Part model, mm, in its own coordinate system. A direction names the side the tool comes from. Round coordinates to 2 decimals unless told otherwise and drop trailing zeros. Write each loop counter-clockwise with the first axis right and the second up, starting at its lowest first coordinate (ties: lowest second). Pieces come first, ordered by that corner, then holes. Notation, with made-up numbers: M -11,-10 L 46,-10 A18 ccw 46,5 Z; hole C -28,89.25 d4. An arc over 180 degrees is marked long. Use a Markdown table: item, result. Add a question column.
1) Which spindle directions (+Z, -Z, +X, -X, +Y, -Y) get a long thin tool onto all of the face, cutting with end or side? Do faces 1 (the face through (16, 4.826, 20)), 2 (the face through (33.018, -22.918, 7.776)). Say none if no direction does.
2) Two-plate mould, pull along X, no slides. Class faces 3 (the face through (33.7, 22.8, 7.8)), 4 (the face through (-14.277, 0.559, 20.398)), 5 (the face through (16, -4.826, 20)), 6 (the face through (11, -11, 40.234)): released by +X, released by -X, zero draft, split by the parting line, or undercut.
3) Slice it at B-B on x = 52. Write the cut outline in (y, z).
4) Slice it at A-A on z = 6.5. Give the number of separate pieces and of enclosed holes in the cut face, plus the area to 3 significant figures.
5) Wall check: probe 1 along Y at (x, z) = (0, 12.5) (1 decimal); probe 2 along X at (y, z) = (1, 8.5); probe 3 along X at (y, z) = (-5, 25). Give the ranges that are in metal, low to high.
6) Drop flat-ended pins along their axis: P1, Ø12, axis at y = -11.5, z = 10, coming from the -X side; P2, Ø6, axis at x = 57.5, y = 12.5, coming from the +Z side; P3, Ø12, axis at x = 60.5, z = 6, coming from the +Y side; P4, Ø16.5, axis at x = 53.975, y = 0, coming from the -Z side. Give the stop position or say it passes through.
```python
from build123d import *

# Parameters (mm, degrees)
F1_DEPTH = 40.2336
F2_R     = 10.16
F3_DEPTH = 15.7734
F5_DEPTH = 40.2346
F6_R     = 3.302


with BuildPart() as f1:
    # F0 (on Top) → F1 (new body)
    with BuildSketch(Plane.XY):
        with BuildLine():
            ThreePointArc((9.512184, -26.945296), (23.327466, -16.503332), (28.575, 0))
            ThreePointArc((28.575, 0), (23.327466, 16.503332), (9.512184, 26.945296))
            ThreePointArc((9.512184, 26.945296), (-28.575, 0), (9.512184, -26.945296))
        make_face()
    extrude(amount=F1_DEPTH)

    # F2 (on Top) + F0 (on Top) → F3 (join)
    with BuildSketch(Plane.XY):
        with BuildLine():
            ThreePointArc((57.191927, -18.776418), (68.538395, -12.280473), (73.025, 0))
            ThreePointArc((73.025, 0), (68.538395, 12.280473), (57.191927, 18.776418))
            ThreePointArc((57.191927, 18.776418), (34.925, 0), (57.191927, -18.776418))
        make_face()
        with Locations((53.975, 0)):
            Circle(F2_R, mode=Mode.SUBTRACT)
    with BuildSketch(Plane.XY):
        with BuildLine():
            ThreePointArc((9.512184, 26.945296), (23.327466, 16.503332), (28.575, 0))
            ThreePointArc((28.575, 0), (23.327466, -16.503332), (9.512184, -26.945296))
            Line((9.512184, -26.945296), (57.191927, -18.776418))
            ThreePointArc((57.191927, -18.776418), (34.925, 0), (57.191927, 18.776418))
            Line((57.191927, 18.776418), (9.512184, 26.945296))
        make_face()
    extrude(amount=F3_DEPTH)

    # F4 (on face) → F5 (cut, through all)
    with BuildSketch(Plane.XY.offset(40.2336)):
        with BuildLine():
            Line((17.889793, 4.826), (13.447765, 4.826))
            ThreePointArc((13.447765, 4.826), (-14.2875, 0), (13.447765, -4.826))
            Line((13.447765, -4.826), (17.889793, -4.826))
            Line((17.889793, -4.826), (17.889793, 4.826))
        make_face()
    extrude(amount=-F5_DEPTH, mode=Mode.SUBTRACT)

    # F6
    f6_edges = [f1.edges().sort_by_distance(p)[0] for p in [
        (-9.512184, 26.945296, 40.2336),
    ]]
    fillet(f6_edges, radius=F6_R)


solid = f1.part
```
Entries:
| question | item | result |
|---|---|---|
| 1 | face 1 | +Z, -Z |
| 1 | face 2 | +Z, -Z, +X, -Y |
| 2 | face 3 | released by +X |
| 2 | face 4 | undercut |
| 2 | face 5 | undercut |
| 2 | face 6 | zero draft |
| 3 | outline | M -19.67,0 L -9.97,0 L -9.97,15.77 L -19.67,15.77 Z; M 9.97,0 L 19.67,0 L 19.67,15.77 L 9.97,15.77 Z |
| 4 | separate pieces | 1 |
| 4 | enclosed holes | 2 |
| 4 | area | 3,440 mm^2 |
| 5 | probe 1 | y = -28.6 to -14.3, 14.3 to 28.6 |
| 5 | probe 2 | x = -28.56 to -14.25, 17.89 to 43.86, 64.09 to 73 |
| 5 | probe 3 | x = -28.13 to -13.38, 13.38 to 28.13 |
| 6 | P1 | stops at x = -28.04 |
| 6 | P2 | stops at z = 15.77 |
| 6 | P3 | stops at y = 19.24 |
| 6 | P4 | passes through |
